from build123d import *

# Parameters (mm, degrees)
SKETCH_1_R          = 1
EXTRUDE_1_DEPTH     = 1.2
SKETCH_2_W          = 1.2
SKETCH_2_H          = 5
EXTRUDE_2_DEPTH     = 8
FILLET_1_R          = 1
SKETCH_4_R          = 1
CUT_EXTRUDE_1_DEPTH = 2


with BuildPart() as part:
    # 草图1 → 凸台-拉伸1 (new body)
    with BuildSketch(Plane.XY):
        with BuildLine():
            Line((1, 0), (7, 0))
            Line((7, 0), (7, 5))
            Line((7, 5), (1, 5))
            ThreePointArc((1, 5), (0.292893219, 4.707106781), (0, 4))
            Line((0, 4), (0, 1))
            ThreePointArc((0, 1), (0.292893219, 0.292893219), (1, 0))
        make_face()
        with Locations((2, 2.5)):
            Circle(SKETCH_1_R, mode=Mode.SUBTRACT)
    extrude(amount=EXTRUDE_1_DEPTH)

    # 草图2 → 凸台-拉伸2 (add)
    with BuildSketch(Plane(origin=(0, 0, 1.2), x_dir=(-1, 0, 0), z_dir=(0, 0, -1))):
        with Locations((-6.4, 2.5)):
            Rectangle(SKETCH_2_W, SKETCH_2_H)
    extrude(amount=-EXTRUDE_2_DEPTH)

    # 圆角1
    fillet_1_edges = [part.edges().sort_by_distance(p)[0] for p in [
        (6.4, 0, 9.2),
        (6.4, 5, 9.2),
    ]]
    fillet(fillet_1_edges, radius=FILLET_1_R)

    # 草图4 → 切除-拉伸1 (cut)
    with BuildSketch(Plane.ZY.offset(-5.8)):
        with Locations((7.2, 2.5)):
            Circle(SKETCH_4_R)
    extrude(amount=-CUT_EXTRUDE_1_DEPTH, mode=Mode.SUBTRACT)


solid = part.part
Geometry check sheet. Reference: the model listing, model coordinates, mm. A direction names the side the tool comes from. Give positions to 0.01 mm unless a question says otherwise; leave off trailing zeros. Write each loop counter-clockwise with the first axis right and the second up, starting at its lowest first coordinate (ties: lowest second). Pieces come first, ordered by that corner, then holes. Notation, with made-up numbers: M -1.75,1 L 54.25,1 A26 cw 54.25,27 Z; hole C 48,-34 d11. An arc over 180 degrees is marked long. One line per question, with ' | ' between items.
1. Cross-section at D-D (x = 4.5). Enter the section's corners in (y, z), plus the area to 3 significant figures.
Ans:
outline: M 0,0 L 5,0 L 5,1.2 L 0,1.2 Z | area: 6.00 mm2
2. Cross-section at A-A (x = 2). Enter the section's corners in (y, z), plus the area to 3 significant figures.
Ans:
outline: M 0,0 L 1.5,0 L 1.5,1.2 L 0,1.2 Z; M 3.5,0 L 5,0 L 5,1.2 L 3.5,1.2 Z | area: 3.60 mm2
3. Cross-section at B-B (y = 2.5). Enter the section's corners in (x, z), plus the area to 3 significant figures.
Ans:
outline: M 0,0 L 1,0 L 1,1.2 L 0,1.2 Z; M 3,0 L 7,0 L 7,6.2 L 5.8,6.2 L 5.8,1.2 L 3,1.2 Z; M 5.8,8.2 L 7,8.2 L 7,9.2 L 5.8,9.2 Z | area: 13.2 mm2
4. Mould release check, pull along Y, two halves, no side actions. Record for faces 3 (the face through (4, 3, 1.2)), 4 (the face through (6.392, 2.8, 8.154)), 5 (the face through (1.263, 3.176, 0.592)), 6 (the face through (6.392, 4.715, 8.899)): released by +Y, released by -Y, zero draft, split by the parting line, or undercut.
Ans:
face 3: zero draft | face 4: undercut | face 5: undercut | face 6: released by +Y
5. Cross-section at C-C (z = 7.2). Enter the section's corners in (x, y), plus the area to 3 significant figures.
Ans:
outline: M 5.8,0 L 7,0 L 7,1.5 L 5.8,1.5 Z; M 5.8,3.5 L 7,3.5 L 7,5 L 5.8,5 Z | area: 3.60 mm2
6. Gauge pin test, flat ends, axial feed: pin 1 (2.5 mm diameter, centred on x = 3, y = 2.5, fed in from +Z); pin 2 (4 mm diameter, centred on x = 2.5, z = 7.5, fed in from -Y); pin 3 (3 mm diameter, centred on y = 4, z = 5.5, fed in from -X). Record the tip position at first contact, or that the pin passes through.
Ans:
pin 1: z = 1.2 | pin 2: through | pin 3: x = 5.8
7. Set-up check for faces 1 (the face through (6, 5, 3)), 2 (the face through (5.8, 2, 5)): record each of +Z, -Z, +X, -X, +Y, -Y from which the full face is reachable in a straight line by a thin tool's end or side.
Ans:
face 1: +Z, -Z, +X, -X, +Y | face 2: +Z, -X, +Y, -Y
8. Scan lines: line 1 along Y through (x, z) = (2, 0.7); line 2 along Z through (x, y) = (0.5, 2.05); line 3 along X through (y, z) = (1.2, 4.5). Record each from-to range of solid material in increasing order. Write a range as from..to.
Ans:
line 1: 0..1.5, 3.5..5 | line 2: 0..1.2 | line 3: 5.8..7
